```python
from build123d import *

# Parameters (mm, degrees)
CROQUIS1_R              = 7.5
SALIENTE_EXTRUIR1_DEPTH = 20
CORTAR_EXTRUIR1_REACH   = 27
CROQUIS2_W              = 10
CROQUIS2_H              = 22.5


with BuildPart() as part:
    # Croquis1 → Saliente-Extruir1 (new body)
    with BuildSketch(Plane(origin=(0, 0, 0), x_dir=(0, 0, -1), z_dir=(1, 0, 0))):
        with BuildLine():
            Line((0, 0), (25, 0))
            Line((25, 0), (25, 17.5))
            ThreePointArc((25, 17.5), (12.5, 30), (0, 17.5))
            Line((0, 17.5), (0, 0))
        make_face()
        with Locations((12.5, 17.5)):
            Circle(CROQUIS1_R, mode=Mode.SUBTRACT)
    extrude(amount=-SALIENTE_EXTRUIR1_DEPTH)

    # Croquis2 → Cortar-Extruir1 (cut, up to next)
    with BuildSketch(Plane.XY, mode=Mode.PRIVATE) as cortar_extruir1_sk1:
        with Locations((-5, 18.75)):
            Rectangle(CROQUIS2_W, CROQUIS2_H)
    cortar_extruir1_tool1 = extrude(cortar_extruir1_sk1.sketch, amount=-CORTAR_EXTRUIR1_REACH, mode=Mode.PRIVATE) & part.part
    add(cortar_extruir1_tool1.solids().sort_by_distance((-5, 18.75, 0))[0], mode=Mode.SUBTRACT)


solid = part.part
```
Design review of the part built by this model. Coordinates are the model's own, in mm. A direction names the side the tool comes from. Round coordinates to 2 decimals unless told otherwise and drop trailing zeros. Write each loop counter-clockwise with the first axis right and the second up, starting at its lowest first coordinate (ties: lowest second). Pieces come first, ordered by that corner, then holes.
Item 1: For faces 1 (the flat face through (-10, 24, -7)), 2 (the flat face through (0, 4, -12)), list the 3-axis set-ups (+Z, -Z, +X, -X, +Y, -Y) from which the entire face can be reached by the end or side of a thin tool; tool diameter is ignored.
Item 2: For probe 1 along Y at (x, z) = (-12.5, -12.5); probe 2 along X at (y, z) = (27, -8.25); probe 3 along Y at (x, z) = (-2.5, -21.25), list the stretches that pass through material, from the lowest coordinate up.
Item 3: The part is to be moulded in two halves that separate along Y. For faces 3 (the flat face through (-12, 7, -25)), 4 (the cylindrical face through (-14.93, 24.936, -11.524)), 5 (the flat face through (-5, 7.5, -12)), say which applies: +Y half, -Y half, draft (parallel to the pull), parting line (faces both ways), or undercut.
Item 4: We need section D-D on x = -2. Write out the cut boundary in (y, z).
Item 5: We need section B-B on y = 14.5. Write out the cut boundary in (x, z).
Item 6: We need section C-C on x = -14.25. Write out the cut boundary in (y, z), and give its area (3 significant figures).
Item 7: Clearance check with flat-ended pins moving along their axes: pin 1 Ø12 at (x, z) = (-11, -19.5) entering from +Y; pin 2 Ø11 at (y, z) = (23, -15.5) entering from +X; pin 3 Ø2 at (x, y) = (-13, 27) entering from -Z. State where each tip first meets the part, or that it passes through.
Item 8: We need section A-A on z = -12.5. Write out the cut boundary in (x, y).
Returned:
1. face 1: +Z, -Z, +X, +Y
1. face 2: +Z, -Z, +X, +Y, -Y
2. probe 1: y = 0 to 10, 25 to 30
2. probe 2: x = -20 to -10
2. probe 3: y = 0 to 7.5
3. face 3: draft
3. face 4: undercut
3. face 5: +Y half
4. outline: (0, -25) - (7.5, -25) - (7.5, 0) - (0, 0) - close
5. outline: (-20, -25) - (-10, -25) - (-10, -19.37) - (-20, -19.37) - close; (-20, -5.63) - (-10, -5.63) - (-10, 0) - (-20, 0) - close
6. outline: (0, -25) - (17.5, -25) arc R12.5 ccw to (17.5, 0) - (0, 0) - close; hole circle Ø15 at (17.5, -12.5)
6. area: 506 mm2
7. pin 1: stops at y = 29.96
7. pin 2: stops at x = -10
7. pin 3: stops at z = -21.67
8. outline: (-20, 0) - (0, 0) - (0, 7.5) - (-10, 7.5) - (-10, 10) - (-20, 10) - close; (-20, 25) - (-10, 25) - (-10, 30) - (-20, 30) - close
